Autodesk Inventor part; units mm, degrees
ref_plane "YZ Plane" through (0, 0, 0) normal (1, 0, 0) x (0, 1, 0)
ref_plane "XZ Plane" through (0, 0, 0) normal (0, 1, 0) x (-1, 0, 0)
ref_plane "XY Plane" through (0, 0, 0) normal (0, 0, 1) x (1, 0, 0)
sketch "Sketch1" plane through (0, 0, 0) normal (0, 0, 1) x (1, 0, 0)
  line L0 (-31.75, 0) -> (31.75, 0)
  line L1 (-31.75, 0) -> (-31.75, 12.7)
  line L2 (-31.75, 12.7) -> (-25.4, 12.7)
  line L3 (-25.4, 12.7) -> (-25.4, 7.9375)
  line L4 (-25.4, 7.9375) -> (-12.7, 7.9375)
  line L5 (-12.7, 7.9375) -> (-12.7, 3.175)
  line L6 (-12.7, 3.175) -> (31.75, 3.175)
  line L7 (31.75, 3.175) -> (31.75, 0)
  point P0 (0, 0)
  point P1 (0, 0)
  dimension "d0" = 25.4
  dimension "d1" = 15.875
  dimension "d2" = 6.35
  dimension "d3" = 6.35
  dimension "d4" = 12.7
  dimension "d5" = 44.45
revolve "Revolution1" add sketch "Sketch1" angle 360 about axis through (-31.75, 0, 0) along (1, 0, 0)
chamfer "Chamfer1" distance 0.7937 angle 45 1 edges at (31.75, -3.175, 0)
properties part number "FE-120-008 Pin" material "Aluminum 6061"
Work out the finished part from the listing and answer in its coordinate system (mm). A direction names the side the tool comes from. Round coordinates to 2 decimals unless told otherwise and drop trailing zeros. Order: outer loops, then holes, each group sorted by start corner. A loop starts at its lowest first (then second) coordinate and runs counter-clockwise, first axis right, second up. Notation, with made-up numbers: M 34,53.25 L 46,53.25 A23 ccw 46,89.25 Z; hole C -32,70 d9. An arc over 180 degrees is marked long. Put each result on its own line as item: value. Start each with the question number.
Q1. Section D-D, the plane y = -4 is taken. Write down the section's boundary in (x, z).
Q2. Flat-ended cylindrical pins translate along their axes: pin 1 (6 mm diameter, centred on x = -0.5, y = -2, fed in from -Z) (3 decimals); pin 2 (8 mm diameter, centred on x = 18.5, z = -3.5, fed in from +Y) (3 decimals); pin 3 (6 mm diameter, centred on y = 7.5, z = -2, fed in from +X). Find the tip coordinate at first contact, or state that the pin passes through.
Q3. Section C-C, the plane x = 9 is taken. Write down the section's boundary in (y, z) (3 decimals).
Q4. Straight lines are drawn through the part: L1, parallel to X at y = 6.75, z = 9; L2, parallel to X at y = -0.25, z = 3.5; L3, parallel to Y at x = -22, z = -0.25. For each, find the intervals that lie inside material, in ascending order. Write a range as [from, to].
Q5. A tool of negligible diameter and unlimited length cuts with its end or side. For faces 1 (the cylindrical face through (-18.96, -1.72, -7.75)), 2 (the flat face through (31.75, 0, 0)), from which of +Z, -Z, +X, -X, +Y, -Y can it reach the whole face along a straight path? Write none if from no direction.
Findings below:
1. outline: M -31.75,-12.05 L -25.4,-12.05 L -25.4,-6.86 L -12.7,-6.86 L -12.7,6.86 L -25.4,6.86 L -25.4,12.05 L -31.75,12.05 Z
2. pin 1: stops at z = -3.175
2. pin 2: stops at y = 3.175
2. pin 3: stops at x = -12.7
3. outline: C 0,0 d6.35
4. L1: x = [-31.75, -25.4]
4. L2: x = [-31.75, -12.7]
4. L3: y = [-7.93, 7.93]
5. face 1: +X
5. face 2: +Z, -Z, +X, +Y, -Y
